from build123d import *

# Parameters (mm, degrees)
SKETCH1_W           = 300
SKETCH1_H           = 300
SKETCH1_W_2         = 200
SKETCH1_H_2         = 200
BOSS_EXTRUDE1_DEPTH = 5
BOSS_EXTRUDE5_DEPTH = 70


with BuildPart() as part:
    # Sketch1 → Boss-Extrude1 (new body)
    with BuildSketch(Plane.XY):
        Rectangle(SKETCH1_W, SKETCH1_H)
        Rectangle(SKETCH1_W_2, SKETCH1_H_2, mode=Mode.SUBTRACT)
    extrude(amount=BOSS_EXTRUDE1_DEPTH)

    # Sketch2 → Boss-Extrude5 (add)
    with BuildSketch(Plane(origin=(0, 0, 0), x_dir=(-1, 0, 0), z_dir=(0, 0, -1))):
        Polygon((-150, -145), (-145, -145), (-145, 145), (-145, 150), (-150, 150), align=None)
        Polygon((145, 145), (145, -145), (150, -145), (150, 150), (145, 150), align=None)
    extrude(amount=BOSS_EXTRUDE5_DEPTH)


solid = part.part
Input: part model. Units: mm. Frame: model coordinates. A direction names the side the tool comes from. Give positions to 0.01 mm unless a question says otherwise; leave off trailing zeros. Order: outer loops, then holes, each group sorted by start corner. A loop starts at its lowest first (then second) coordinate and runs counter-clockwise, first axis right, second up.
Q1. Ray query, probe 1 along X at (y, z) = (116, -50.5); probe 2 along X at (y, z) = (66, 1); probe 3 along Z at (x, y) = (-40.5, 121). Return the intervals inside material, ascending.
Checked values:
probe 1: x = -150 to -145, 145 to 150
probe 2: x = -150 to -100, 100 to 150
probe 3: z = 0 to 5
Q2. Draft query along X for faces 3 (the flat face through (-2, 102, 5)), 4 (the flat face through (150, 2, -32)), 5 (the flat face through (-145, 5, -35)). Return one class per face: +X half, -X half, draft (parallel to the pull), parting line (faces both ways), or undercut.
Checked values:
face 3: draft
face 4: +X half
face 5: undercut
Q3. Section D-D on y = -111. Output: boundary loops of the cut face in (x, z), and give its area (3 significant figures).
Checked values:
outline: (-150, -70) - (-145, -70) - (-145, 0) - (145, 0) - (145, -70) - (150, -70) - (150, 5) - (-150, 5) - close
area: 2,200 mm2
Q4. Set-up query: faces 1 (the flat face through (145, 0, -35)), 2 (the flat face through (-150, -2, -33)). Return all of +Z, -Z, +X, -X, +Y, -Y with unobstructed straight access to the full face (end or side cutting, diameter ignored); none if empty.
Checked values:
face 1: -Z, +Y, -Y
face 2: +Z, -Z, -X, +Y, -Y
Q5. Section C-C on x = -47. Output: boundary loops of the cut face in (y, z), and give its area (3 significant figures).
Checked values:
outline: (-150, 0) - (-100, 0) - (-100, 5) - (-150, 5) - close; (100, 0) - (150, 0) - (150, 5) - (100, 5) - close
area: 500 mm2
Q6. Section A-A on z = -18. Output: boundary loops of the cut face in (x, y), and give its area (3 significant figures).
Checked values:
outline: (-150, -145) - (-145, -145) - (-145, 150) - (-150, 150) - close; (145, -145) - (150, -145) - (150, 150) - (145, 150) - close
area: 2,950 mm2
Q7. Contact query for a flat-ended pin moving along its axis: pin 1 Ø4 at (x, z) = (147, -42) entering from -Y. Output: stop coordinate, or through.
Checked values:
pin 1: stops at y = -145
Q8. Section B-B on y = -54. Output: boundary loops of the cut face in (x, z), and give its area (3 significant figures).
Checked values:
outline: (-150, -70) - (-145, -70) - (-145, 0) - (-100, 0) - (-100, 5) - (-150, 5) - close; (100, 0) - (145, 0) - (145, -70) - (150, -70) - (150, 5) - (100, 5) - close
area: 1,200 mm2
